The figure shows three views and two pictorial views of one solid part (mm, origin at its lowest corner). Answer the questions. A direction names the side the tool comes from. Coordinates: 2 decimals unless noted, no trailing zeros. Loops run counter-clockwise (first coordinate to the right, second up) from the corner with the lowest first, then second, coordinate; pieces in that order, holes last. Notation, with made-up numbers: M -31.5,55 L -22.5,55 A24 ccw -22.5,78 Z; hole C 65,11.5 d3. An arc over 180 degrees is marked long. Answer as a JSON object with one key per item and string values. Group by question number.
1. For the marked faces 1, 2 and 3, determine the directions among +Z, -Z, +X, -X, +Y, -Y from which every point of the face is accessible in a straight line to the end or side of a thin tool.
2. A cutting plane is placed at B-B on x = 87. Give the vertices of the cut face in (y, z).
3. Given pin 1 (9 mm diameter, centred on x = 33, y = 22, fed in from -Z); pin 2 (9 mm diameter, centred on x = 90, z = 30, fed in from -Y); pin 3 (8 mm diameter, centred on y = 4, z = 25.5, fed in from +X); pin 4 (1.5 mm diameter, centred on x = 14, z = 10, fed in from +Y), each flat-ended and moving along its own axis, determine where each tip first touches the part or whether it passes through.
4. A cutting plane is placed at C-C on z = 31.5. Give the vertices of the cut face in (x, y).
5. Straight lines are drawn through the part: L1, parallel to Z at x = 69.5, y = 24.5; L2, parallel to X at y = 19, z = 30; L3, parallel to X at y = 19.5, z = 30. For each, find the intervals that lie inside material, in ascending order.
6. Determine the mould class of the marked faces 4, 5 and 6 for opening direction X: released by +X, released by -X, zero draft, split by the parting line, or undercut.
7. A cutting plane is placed at D-D on x = 13. Give the vertices of the cut face in (y, z), and give its area (3 significant figures).
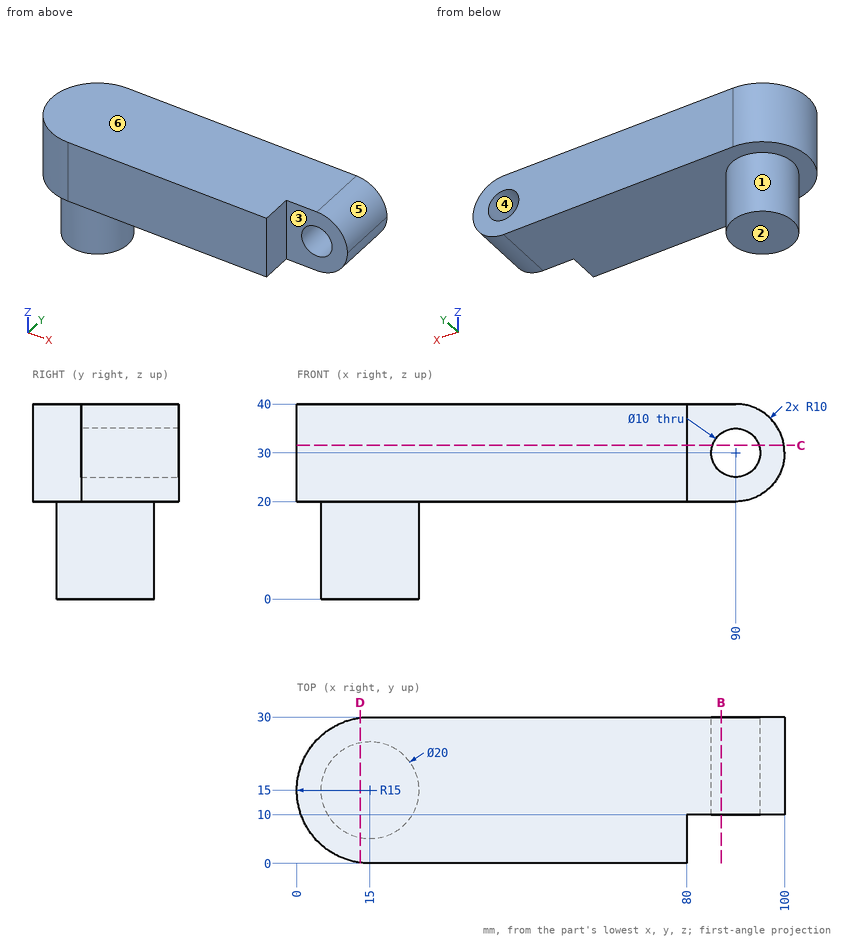
From the geometry:
{
 "1": {"face 1": "-Z", "face 2": "-Z, +X, -X, +Y, -Y", "face 3": "+Z, -Z, +X, -Y"},
 "2": {"outline": "M 10,20 L 30,20 L 30,26 L 10,26 Z; M 10,34 L 30,34 L 30,40 L 10,40 Z"},
 "3": {"pin 1": "stops at z = 20", "pin 2": "passes through", "pin 3": "stops at x = 80", "pin 4": "stops at y = 25"},
 "4": {"outline": "M 15,0 L 80,0 L 80,10 L 85.23,10 L 85.23,30 L 15,30 A15 ccw Z; M 94.77,10 L 99.89,10 L 99.89,30 L 94.77,30 Z"},
 "5": {"L1": "z = 20 to 40", "L2": "x = 0.54 to 85, 95 to 100", "L3": "x = 0.69 to 85, 95 to 100"},
 "6": {"face 4": "undercut", "face 5": "released by +X", "face 6": "zero draft"},
 "7": {"outline": "M 0.13,20 L 5.2,20 L 5.2,0 L 24.8,0 L 24.8,20 L 29.87,20 L 29.87,40 L 0.13,40 Z", "area": "987 mm²"}
}
